```python
from build123d import *

# Parameters (mm, degrees)
FILLET1_R       = 0.25
SKETCH3_W       = 1.42
SKETCH3_H       = 6.7
SKETCH4_W       = 1.42
SKETCH4_H       = 3.249815392
RECPAT_COUNT    = 2
RECPAT_ANGLE    = 90
THDSCHPAT_COUNT = 15
THDSCHPAT_PITCH = 1


with BuildPart() as part:
    # BodySke → Base-Revolve (revolve)
    with BuildSketch(Plane.XY):
        with BuildLine():
            Line((4.6, 3), (4.6, 6))
            Line((4.6, 6), (2.274716834, 6))
            ThreePointArc((2.274716834, 6), (2.026424569, 5.939532013), (1.833738725, 5.77167019))
            ThreePointArc((1.833738725, 5.77167019), (0.469454036, 3.027985077), (0, 0))
            Line((0, 0), (20.6, 0))
            Line((20.6, 0), (20.6, 3))
            Line((20.6, 3), (4.6, 3))
        make_face()
    revolve(axis=Axis((-25.4, 0, 0), (1, 0, 0)))

    # Fillet1
    fillet1_edges = [part.edges().sort_by_distance(p)[0] for p in [
        (4.6, -3, 0),
    ]]
    fillet(fillet1_edges, radius=FILLET1_R)

    # Sketch3 → Recess section 0
    with BuildSketch(Plane(origin=(0, 0, 0), x_dir=(0, 0, -1), z_dir=(1, 0, 0))):
        Rectangle(SKETCH3_W, SKETCH3_H)
    # Sketch4 → Recess section 1
    with BuildSketch(Plane(origin=(3.46, 0, 0), x_dir=(0, 0, -1), z_dir=(1, 0, 0))):
        Rectangle(SKETCH4_W, SKETCH4_H)
    recess = loft(mode=Mode.SUBTRACT)

    # RecPat: Recess ×2 about axis
    recpat_axis = Axis((0, 0, 0), (1, 0, 0))
    for i in range(1, RECPAT_COUNT):
        add(recess.rotate(recpat_axis, i * RECPAT_ANGLE / (RECPAT_COUNT - 1)), mode=Mode.SUBTRACT)

    # RecCorSke → RecessCore (revolve, cut)
    with BuildSketch(Plane.XY):
        Polygon((0, 0), (0, 1.522446769), (3.46, 1.2805), (3.876059671, 0), align=None)
    revolve(axis=Axis((-3.175, 0, 0), (1, 0, 0)), mode=Mode.SUBTRACT)

    # ThdSchSke → ThreadSchematic (revolve, cut)
    with BuildSketch(Plane.XY):
        Polygon((6.6, -2.4455), (6.21173492, -3), (6.21173492, -3.75), (6.98826508, -3.75), (6.98826508, -3), align=None)
    threadschematic = revolve(axis=Axis((-3.175, 0, 0), (1, 0, 0)), mode=Mode.SUBTRACT)

    # ThdSchPat: ThreadSchematic ×15
    with Locations(*[(i * THDSCHPAT_PITCH, 0, 0) for i in range(1, THDSCHPAT_COUNT)]):
        add(threadschematic, mode=Mode.SUBTRACT)


solid = part.part
```
Geometry check sheet. Reference: the model listing, model coordinates, mm. A direction names the side the tool comes from. Coordinates: 2 decimals unless noted, no trailing zeros.
Item 1: Tool access check on faces 1 (the flat face through (20.6, 0, 0)), 2 (the flat face through (1.998, 0.01, 2.354)). Record the directions out of +Z, -Z, +X, -X, +Y, -Y that give a thin tool (end or side, any length) a straight path to the whole face; none if there is none.
Item 2: Depth check by flat-ended pin: pin 1 (0.6 mm diameter, centred on y = 1, z = 0, fed in from -X); pin 2 (0.6 mm diameter, centred on y = 0, z = -1.5, fed in from -X); pin 3 (2 mm diameter, centred on x = 14.5, z = 1.5, fed in from -Y). Enter the tip coordinate at first touch or a pass-through.
Item 3: Scan lines: line 1 along Z through (x, y) = (1, 0); line 2 along X through (y, z) = (1.5, 0.25); line 3 along X through (y, z) = (2.25, 3.5). Record each from-to range of solid material in increasing order.
Item 4: Section check A-A (y = 2.75). Count the separate pieces of the cut face and the enclosed holes in it, plus the area to 3 significant figures.
Check sheet entries:
1. face 1: +Z, -Z, +X, +Y, -Y
1. face 2: -X
2. pin 1: stops at x = 3.46
2. pin 2: stops at x = 3.11
2. pin 3: stops at y = -2.95
3. line 1: z = -4.36 to -2.85, 2.85 to 4.36
3. line 2: x = 3.46 to 20.6
3. line 3: x = 0.91 to 4.6
4. separate pieces: 15
4. enclosed holes: 0
4. area: 57.7 mm2
